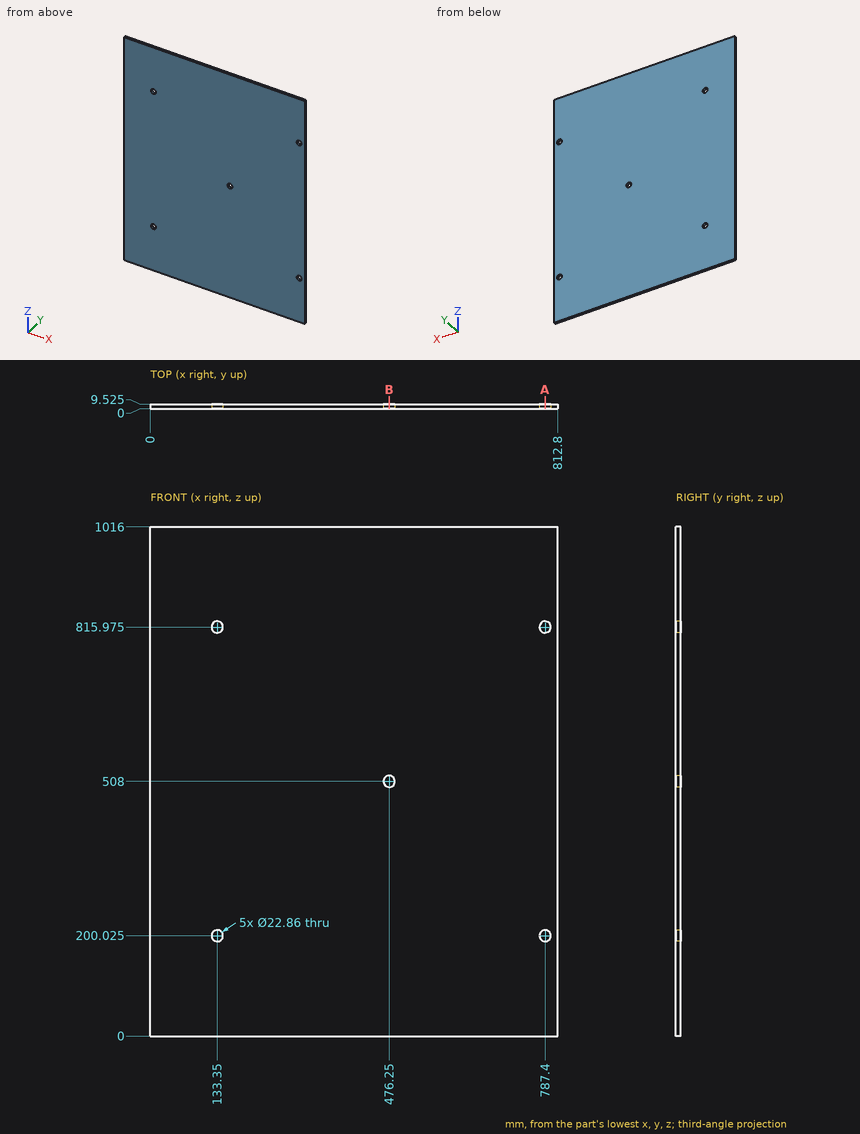
Here's the drawing with two shaded views (mm, measured from the low corner). I have some questions. Give positions to 0.01 mm unless a question says otherwise; leave off trailing zeros. Order: outer loops, then holes, each group sorted by start corner. A loop starts at its lowest first (then second) coordinate and runs counter-clockwise, first axis right, second up.
Q1. Suppose I cut it at B-B, the plane x = 476.25. Write out the boundary of the cut face in (y, z) (3 decimals), and give its area (3 significant figures).
Q2. If I drill on line 1 along Z through (x, y) = (787.4, 4.25) (3 decimals); line 2 along X through (y, z) = (6.75, 508); line 3 along Z through (x, y) = (476.25, 5), over which ranges is the centre line in solid material (lowest first)?
Q3. Suppose I cut it at A-A, the plane x = 787.4. Write out the boundary of the cut face in (y, z) (3 decimals), and give its area (3 significant figures).
Solution:
1. outline: (0, 0) - (9.525, 0) - (9.525, 496.57) - (0, 496.57) - close; (0, 519.43) - (9.525, 519.43) - (9.525, 1016) - (0, 1016) - close
1. area: 9,460 mm2
2. line 1: z = 0 to 188.595, 211.455 to 804.545, 827.405 to 1016
2. line 2: x = 0 to 464.82, 487.68 to 812.8
2. line 3: z = 0 to 496.57, 519.43 to 1016
3. outline: (0, 0) - (9.525, 0) - (9.525, 188.595) - (0, 188.595) - close; (0, 211.455) - (9.525, 211.455) - (9.525, 804.545) - (0, 804.545) - close; (0, 827.405) - (9.525, 827.405) - (9.525, 1016) - (0, 1016) - close
3. area: 9,240 mm2
